Can you work these out from the model? Positions are in its coordinate system, mm. Round coordinates to 2 decimals unless told otherwise and drop trailing zeros. Write each loop counter-clockwise with the first axis right and the second up, starting at its lowest first coordinate (ties: lowest second). Pieces come first, ordered by that corner, then holes. Notation, with made-up numbers: M -36,-20 L 6,-20 A24 ccw 6,0 Z; hole C -5,44.5 d3. An arc over 180 degrees is marked long. Answer in a Markdown table with one row per item. Add a question column.
(1) Suppose I cut it at A-A, the plane x = 0. Write out the boundary of the cut face in (y, z), then the cut area to 3 significant figures.
(2) I'm going to push a flat-ended pin straight in: pin 1 (1.5 mm diameter, centred on x = -1, z = -19, fed in from -Y). Where does the tip first touch, or does it pass through?
(3) Suppose I cut it at B-B, the plane z = 4. Write out the boundary of the cut face in (x, y), then the cut area to 3 significant figures.
(4) If I drill on probe 1 along Y at (x, z) = (0.4, 25.5), over which ranges is the centre line in solid material (lowest first)?
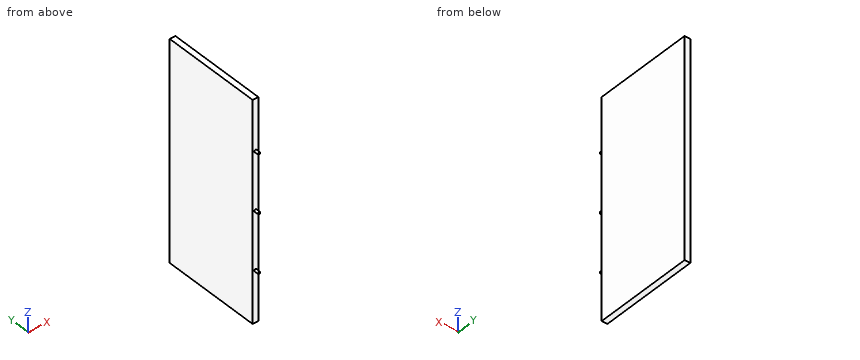
Autodesk Inventor part; units mm, degrees
ref_plane "YZ Plane" through (0, 0, 0) normal (1, 0, 0) x (0, 1, 0)
ref_plane "XZ Plane" through (0, 0, 0) normal (0, 1, 0) x (-1, 0, 0)
ref_plane "XY Plane" through (0, 0, 0) normal (0, 0, 1) x (1, 0, 0)
sketch "Sketch1" plane through (0, 0, 0) normal (0, 1, 0) x (-1, 0, 0)
  line L0 (2, 77) -> (-2, 77)
  line L1 (-2, 77) -> (-2, -77)
  line L2 (-2, -77) -> (2, -77)
  line L3 (2, -77) -> (2, 77)
  line L4 (2, 77) -> (-2, -77) construction
  line L5 (-2, 77) -> (2, -77) construction
  circle A0 centre (0, -41) radius 0.85
  circle A1 centre (0, 0) radius 0.85
  circle A2 centre (0, 41) radius 0.85
  point P0 (0, 0)
  dimension "d0" = 154
  dimension "d1" = 4
  dimension "d2" = 1.7
  dimension "d3" = 2
  dimension "d4" = 36
  dimension "d5" = 1.7
  dimension "d6" = 2
  dimension "d8" = 77
  dimension "d9" = 1.7
  dimension "d10" = 2
  dimension "d11" = 118
extrude "MainBody" add sketch "Sketch1" along normal blind 70
sketch "Sketch2" plane through (0, 0, 0) normal (0, -1, 0) x (1, 0, 0)
  circle A0 centre (0, 0) radius 0.85
extrude "MiddlePole" add sketch "Sketch2" along normal blind 3 and the other way blind 70
sketch "Sketch3" plane through (0, 0, 0) normal (0, -1, 0) x (1, 0, 0)
  circle A0 centre (0, 41) radius 0.85
  circle A1 centre (0, 41) radius 0.85
  point P0 (0, 0)
extrude "UpperPole" add sketch "Sketch3" along normal blind 3 and the other way blind 70
sketch "Sketch4" plane through (0, 0, 0) normal (0, -1, 0) x (1, 0, 0)
  circle A0 centre (0, -41) radius 0.85
  point P0 (0, 0)
extrude "LowerPole" add sketch "Sketch4" along normal blind 3 and the other way blind 70
properties part number "DindingKargoKananKiri"
Calculated:
| question | item | result |
|---|---|---|
| 1 | outline | M -3,-41.85 L 0,-41.85 L 0,-77 L 70,-77 L 70,77 L 0,77 L 0,41.85 L -3,41.85 L -3,40.15 L 0,40.15 L 0,0.85 L -3,0.85 L -3,-0.85 L 0,-0.85 L 0,-40.15 L -3,-40.15 Z |
| 1 | area | 10,800 mm² |
| 2 | pin 1 | y = 0 |
| 3 | outline | M -2,0 L 2,0 L 2,70 L -2,70 Z |
| 3 | area | 280 mm² |
| 4 | probe 1 | 0 to 70 |
